Answer from the drawing. Dimensions are ordinates in mm from the lowest x, y and z of the part. Coordinates: 2 decimals unless noted, no trailing zeros. Write each loop counter-clockwise with the first axis right and the second up, starting at its lowest first coordinate (ties: lowest second). Pieces come first, ordered by that corner, then holes.
(1) Section C-C on z = 12.75 is taken. Write down the section's boundary in (x, y).
(2) Given pin 1 (5 mm diameter, centred on x = 10.105, z = 7.5, fed in from +Y), flat-ended and moving along its own axis, determine where the tip first touches the part or whether it passes through.
(3) Section B-B on y = 2.7 is taken. Write down the section's boundary in (x, z) (3 decimals), then the cut area to 3 significant figures.
(4) The mould has two halves that part along X. Classify the marked faces 1, 2 and 3: +X half, -X half, draft (parallel to the pull), parting line (faces both ways), or undercut.
(5) Section A-A on z = 7.5 is taken. Write down the section's boundary in (x, y) (3 decimals), then the cut area to 3 significant figures.
(6) Section D-D on y = 0.6 is taken. Write down the section's boundary in (x, z) (3 decimals).
(7) Find the intervals of material crossed by probe 1 along Z at (x, y) = (13.75, 0.95); probe 2 along X at (y, z) = (2.2, 4); probe 3 along Z at (x, y) = (12, 2.35), in increasing order.
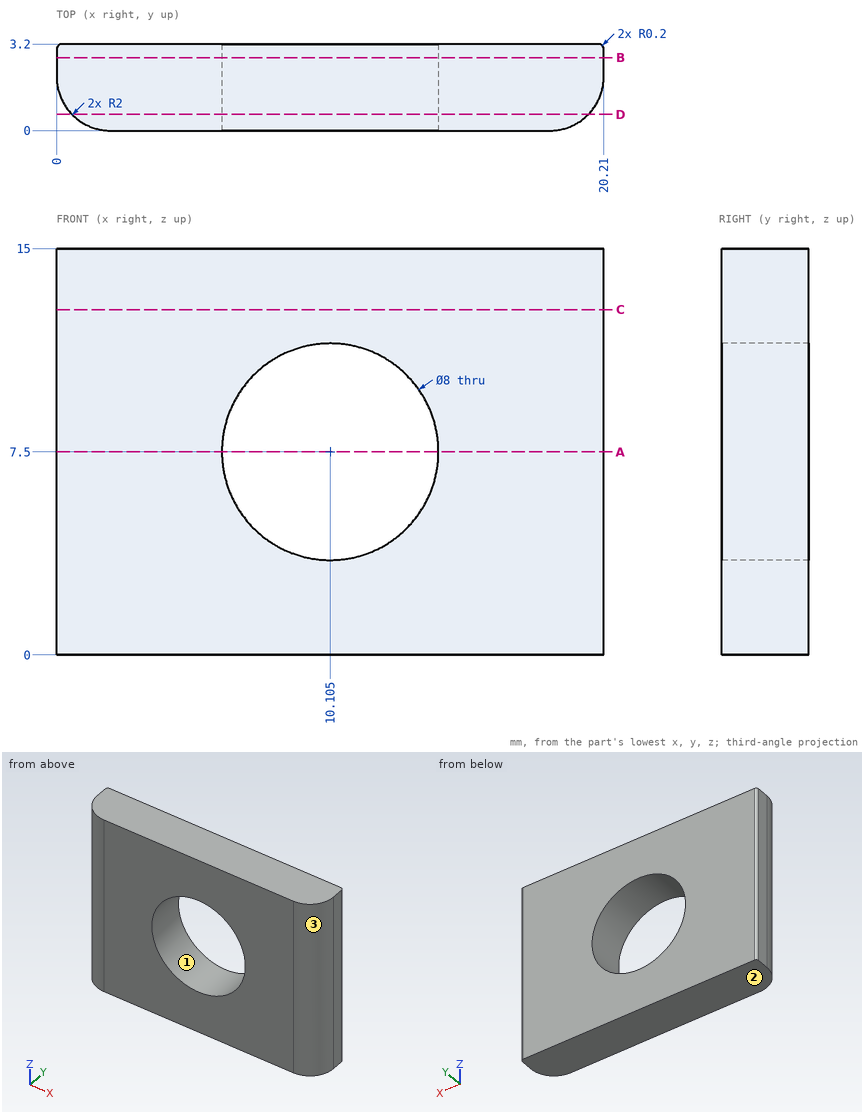
Response:
1. outline: (0, 2) arc R2 ccw to (2, 0) - (18.21, 0) arc R2 ccw to (20.21, 2) - (20.21, 3) arc R0.2 ccw to (20.01, 3.2) - (0.2, 3.2) arc R0.2 ccw to (0, 3) - close
2. pin 1: passes through
3. outline: (0, 0) - (20.21, 0) - (20.21, 15) - (0, 15) - close; hole circle Ø8 at (10.105, 7.5)
3. area: 253 mm2
4. face 1: undercut
4. face 2: draft
4. face 3: +X half
5. outline: (0, 2) arc R2 ccw to (2, 0) - (6.105, 0) - (6.105, 3.2) - (0.2, 3.2) arc R0.2 ccw to (0, 3) - close; (14.105, 0) - (18.21, 0) arc R2 ccw to (20.21, 2) - (20.21, 3) arc R0.2 ccw to (20.01, 3.2) - (14.105, 3.2) - close
5. area: 37.3 mm2
6. outline: (0.572, 0) - (19.638, 0) - (19.638, 15) - (0.572, 15) - close; hole circle Ø8 at (10.105, 7.5)
7. probe 1: z = 0 to 5.85, 9.15 to 15
7. probe 2: x = 0 to 8.17, 12.04 to 20.21
7. probe 3: z = 0 to 3.98, 11.02 to 15
